from build123d import *

# Parameters (mm, degrees)
SKETCH1_W           = 150
SKETCH1_H           = 30
BOSS_EXTRUDE1_DEPTH = 30
SHELL1_T            = -3
SKETCH2_R           = 5
CUT_EXTRUDE1_DEPTH  = 30
SKETCH3_R           = 4
CUT_EXTRUDE2_DEPTH  = 36


with BuildPart() as part:
    # Sketch1 → Boss-Extrude1 (new body)
    with BuildSketch(Plane.XY):
        Rectangle(SKETCH1_W, SKETCH1_H)
    extrude(amount=BOSS_EXTRUDE1_DEPTH)

    # Shell1
    shell1_openings = [part.faces().sort_by_distance(p)[0] for p in [
        (-75, 0, 15),
        (75, 0, 15),
    ]]
    offset(amount=SHELL1_T, openings=shell1_openings, kind=Kind.INTERSECTION)

    # Sketch2 → Cut-Extrude1 (cut)
    with BuildSketch(Plane.XY.offset(30)):
        Circle(SKETCH2_R)
    extrude(amount=-CUT_EXTRUDE1_DEPTH, mode=Mode.SUBTRACT)

    # Sketch3 → Cut-Extrude2 (cut)
    with BuildSketch(Plane(origin=(0, 15, 0), x_dir=(1, 0, 0), z_dir=(0, 1, 0))):
        with Locations((-55, -15)):
            Circle(SKETCH3_R)
        with Locations((55, -15)):
            Circle(SKETCH3_R)
    extrude(amount=-CUT_EXTRUDE2_DEPTH, mode=Mode.SUBTRACT)


solid = part.part
Verification items for the finished model (mm, model axes). A direction names the side the tool comes from. Coordinates: 2 decimals unless noted, no trailing zeros. Order: outer loops, then holes, each group sorted by start corner. A loop starts at its lowest first (then second) coordinate and runs counter-clockwise, first axis right, second up. Notation, with made-up numbers: M -7.75,-8.5 L 48.25,-8.5 A24 ccw 48.25,3.5 Z; hole C 59.5,1 d2. An arc over 180 degrees is marked long. Write each question's results on one line, items separated by ' | '.
1) Section check B-B on y = 7.25. Record the cut outline in (x, z).
Solved:
outline: M -75,0 L 75,0 L 75,3 L -75,3 Z; M -75,27 L 75,27 L 75,30 L -75,30 Z
2) Section check C-C on z = 15. Record the cut outline in (x, y).
Solved:
outline: M -75,-15 L -59,-15 L -59,-12 L -75,-12 Z; M -75,12 L -59,12 L -59,15 L -75,15 Z; M -51,-15 L 51,-15 L 51,-12 L -51,-12 Z; M -51,12 L 51,12 L 51,15 L -51,15 Z; M 59,-15 L 75,-15 L 75,-12 L 59,-12 Z; M 59,12 L 75,12 L 75,15 L 59,15 Z
3) Section check A-A on x = 0. Record the cut outline in (y, z).
Solved:
outline: M -15,0 L -5,0 L -5,3 L -12,3 L -12,27 L -5,27 L -5,30 L -15,30 Z; M 5,0 L 15,0 L 15,30 L 5,30 L 5,27 L 12,27 L 12,3 L 5,3 Z
4) Access from +Z, -Z, +X, -X, +Y, -Y to the whole of each face (thin tool, end or side, straight path). Record for faces 1 (the face through (-1, 6, 3)), 2 (the face through (-1.08, -4.88, 1.52)).
Solved:
face 1: +X, -X | face 2: +Z, -Z
5) Section check D-D on x = -37. Record the cut outline in (y, z).
Solved:
outline: M -15,0 L 15,0 L 15,30 L -15,30 Z; hole M -12,3 L 12,3 L 12,27 L -12,27 Z
6) Release check for a two-part mould opening along Z. For faces 3 (the face through (-1, 12, 15)), 4 (the face through (-1, -15, 15)), 5 (the face through (-51.185, -13.479, 13.799)), 6 (the face through (-1, 7, 30)) record: pulls with the +Z half, pulls with the -Z half, needs draft (parallel to the pull), parting line crosses it, or undercut.
Solved:
face 3: undercut | face 4: needs draft | face 5: undercut | face 6: pulls with the +Z half
7) Scan lines: line 1 along X through (y, z) = (-12.9, 15); line 2 along Z through (x, y) = (40, -2); line 3 along Y through (x, z) = (-39, 5). Record each from-to range of solid material in increasing order. Write a range as [from, to].
Solved:
line 1: x = [-75, -59], [-51, 51], [59, 75] | line 2: z = [0, 3], [27, 30] | line 3: y = [-15, -12], [12, 15]
